from build123d import *

# Parameters (mm, degrees)
ESQUISSE1_R             = 17
BOSS_EXTRU_1_DEPTH      = 96
ESQUISSE2_W             = 70
ESQUISSE2_H             = 58.5
BOSS_EXTRU_3_DEPTH      = 65
ESQUISSE6_R             = 18
BOSS_EXTRU_4_DEPTH      = 144
ESQUISSE7_W             = 70
ESQUISSE7_H             = 18
ENL_V_MAT_EXTRU_1_DEPTH = 5.5
ESQUISSE8_W             = 70
ESQUISSE8_H             = 1.25
ENL_V_MAT_EXTRU_2_DEPTH = 2
ESQUISSE9_R             = 2.5
BOSS_EXTRU_5_DEPTH      = 120
CONG_1_R                = 1


with BuildPart() as part:
    # Esquisse1 → Boss.-Extru.1 (new body)
    with BuildSketch(Plane(origin=(0, 0, 0), x_dir=(0, 0, -1), z_dir=(1, 0, 0))):
        Circle(ESQUISSE1_R)
    extrude(amount=BOSS_EXTRU_1_DEPTH)

    # Esquisse2 → Boss.-Extru.3 (add)
    with BuildSketch(Plane(origin=(96, 0, 0), x_dir=(0, 0, -1), z_dir=(1, 0, 0))):
        with Locations((0, -6.25)):
            Rectangle(ESQUISSE2_W, ESQUISSE2_H)
    extrude(amount=BOSS_EXTRU_3_DEPTH)

    # Esquisse6 → Boss.-Extru.4 (add)
    with BuildSketch(Plane(origin=(88.685287476, 51.850448358, 0), x_dir=(0, 0, -1), z_dir=(0.8632812499999999, 0.5047231750162041, 0))):
        with Locations(Location((0, -60.062057827, 0), (0, 0, 90))):
            Circle(ESQUISSE6_R)
    extrude(amount=-BOSS_EXTRU_4_DEPTH)

    # Esquisse7 → Enlèv. mat.-Extru.1 (cut)
    with BuildSketch(Plane(origin=(161, 0, 0), x_dir=(0, 0, -1), z_dir=(1, 0, 0))):
        with Locations((0, -26.5)):
            Rectangle(ESQUISSE7_W, ESQUISSE7_H)
    extrude(amount=-ENL_V_MAT_EXTRU_1_DEPTH, mode=Mode.SUBTRACT)

    # Esquisse8 → Enlèv. mat.-Extru.2 (cut)
    with BuildSketch(Plane(origin=(155.5, 0, 0), x_dir=(0, 0, -1), z_dir=(1, 0, 0))):
        with Locations((0, -34.875)):
            Rectangle(ESQUISSE8_W, ESQUISSE8_H)
    extrude(amount=-ENL_V_MAT_EXTRU_2_DEPTH, mode=Mode.SUBTRACT)

    # Esquisse9 → Boss.-Extru.5 (add)
    with BuildSketch(Plane(origin=(-35.627212524, -20.829688844, 0), x_dir=(0, 0, 1), z_dir=(-0.8632812499999999, -0.5047231750162042, 0))):
        with Locations((-19.5, -60.062057827)):
            Circle(ESQUISSE9_R)
    extrude(amount=-BOSS_EXTRU_5_DEPTH)

    # Congé1
    cong_1_edges = [part.edges().sort_by_distance(p)[0] for p in [
        (44.859518924, -41.124048908, -17.897435897),
        (45.827981076, -45.003192614, -17.897435897),
    ]]
    fillet(cong_1_edges, radius=CONG_1_R)


solid = part.part
Can you work these out from the model? Positions are in its coordinate system, mm. A direction names the side the tool comes from. Coordinates: 2 decimals unless noted, no trailing zeros. Loops run counter-clockwise (first coordinate to the right, second up) from the corner with the lowest first, then second, coordinate; pieces in that order, holes last. Notation, with made-up numbers: (-7, 18) - (51, 18) arc R21 ccw to (51, 26) - close; hole circle Ø3 at (20, 39). An arc over 180 degrees is marked (long way). Answer as a JSON object with one key per item and string values. Group by question number.
Item 1: If we section it at A-A (y = 0): List the corners of the cut face in (x, z) for me.
Item 2: If we section it at B-B (z = -27): List the corners of the cut face in (x, y) for me, plus the area to 3 significant figures.
Item 3: If we section it at D-D (z = 0): List the corners of the cut face in (x, y) for me, plus the area to 3 significant figures.
Item 4: If I drill on L1, parallel to Y at x = 109, z = -19.5; L2, parallel to X at y = 4, z = -9.5; L3, parallel to X at y = 16.5, z = -15, over which ranges is the centre line in solid material (lowest first)? Write a range as from..to.
Item 5: On a 3-axis mill with a long thin cutter (end or side, diameter ignored), from which of +Z, -Z, +X, -X, +Y, -Y can I reach the whole of each face in a straight line? I mean faces 1 (the face through (155.5, -26, 0)), 2 (the face through (47.328, 16.855, 2.213)), 3 (the face through (41.559, -57.334, 14.685)). Say none if no direction works.
Item 6: If we section it at C-C (x = 143.5): List the corners of the cut face in (y, z) for me, plus the area to 4 significant figures.
Item 7: For pin 1 (6 mm diameter, centred on x = 29, y = -5.5, fed in from +Z); pin 2 (1.6 mm diameter, centred on x = 155, z = 17, fed in from -Y); pin 3 (1.6 mm diameter, centred on x = 158.5, z = -6.5, fed in from -Y); pin 4 (18.5 mm diameter, centred on y = -23.5, z = -12.5, fed in from +X), each with a flat end and sliding along its axis, tell me the tip position at first contact or that it passes through.
Item 8: If we mould it in two halves opening along X, with no side actions, what happens to faces 4 (the face through (0, 0, 0)), 5 (the face through (124, -35.5, 0)), 6 (the face through (161, 3, 0)), 7 (the face through (45.2, -43.1, -22))? For each: released by +X, released by -X, zero draft, split by the parting line, or undercut.
Returned:
{
 "1": {"outline": "(0, -17) - (96, -17) - (96, -35) - (161, -35) - (161, 35) - (96, 35) - (96, 17) - (0, 17) - close"},
 "2": {"outline": "(96, -35.5) - (153.5, -35.5) - (153.5, -34.25) - (155.5, -34.25) - (155.5, -17.5) - (161, -17.5) - (161, 23) - (96, 23) - close", "area": "3,700 mm²"},
 "3": {"outline": "(-14.4, -57.14) - (3.77, -88.22) - (96, -34.3) - (96, -35.5) - (153.5, -35.5) - (153.5, -34.25) - (155.5, -34.25) - (155.5, -17.5) - (161, -17.5) - (161, 23) - (96, 23) - (96, 17) - (0, 17) - (0, -17) - (54.26, -17) - close", "area": "10,700 mm²"},
 "4": {"L1": "y = -35.5..23", "L2": "x = 0..161", "L3": "x = 96..161"},
 "5": {"face 1": "+Z, -Z, +X, -Y", "face 2": "-X", "face 3": "none"},
 "6": {"outline": "(-35.5, -35) - (23, -35) - (23, 35) - (-35.5, 35) - close", "area": "4,095 mm²"},
 "7": {"pin 1": "stops at z = 16.82", "pin 2": "stops at y = -34.25", "pin 3": "stops at y = -17.5", "pin 4": "stops at x = 161"},
 "8": {"face 4": "released by -X", "face 5": "zero draft", "face 6": "released by +X", "face 7": "undercut"}
}
